Here's how the part is built. I have some questions about the finished solid (model axes, mm). Round coordinates to 2 decimals unless told otherwise and drop trailing zeros. Write each loop counter-clockwise with the first axis right and the second up, starting at its lowest first coordinate (ties: lowest second). Pieces come first, ordered by that corner, then holes. Notation, with made-up numbers: M 17.5,84.5 L 53.5,84.5 A30 ccw 53.5,122.5 Z; hole C -17,80 d4. An arc over 180 degrees is marked long. Use a Markdown table: item, result. Add a question column.
```python
from build123d import *

# Parameters (mm, degrees)
F0_R     = 3.6643363337
F0_R_2   = 12.1990402392
F1_DEPTH = 6.35


# Not quite as in the source:
# - a feature names something its author has since deleted; it is built from what else it names


with BuildPart() as f1:
    # F0 (on Top) → F1 (new body)
    with BuildSketch(Plane.XY):
        Polygon((4.9436837435, 38.7340840895), (-45.8563162565, 38.7340840895), (-45.8563162565, -50.1659159105), (4.9436837435, -50.1659159105), (30.3436837435, -50.1659159105), (55.7436837435, -50.1659159105), (55.7436837435, -5.7159159105), (55.7436837435, 38.7340840895), (30.3436837435, 38.7340840895), align=None)
        with Locations((43.0436837435, -27.9409159105)):
            Circle(F0_R, mode=Mode.SUBTRACT)
        with Locations((-20.4563162565, -5.7159159105)):
            Circle(F0_R_2, mode=Mode.SUBTRACT)
        with Locations((43.0436837435, 16.5090840895)):
            Circle(F0_R, mode=Mode.SUBTRACT)
    extrude(amount=F1_DEPTH)


solid = f1.part
```
Item 1: If we mould it in two halves opening along Y, with no side actions, what happens to faces 1 (the face through (-32.644, -5.18, 3.131)), 2 (the face through (44.735, 13.258, 3.131)), 3 (the face through (6, 38.734, 3)), 4 (the face through (4, -5, 0))? For each: +Y half, -Y half, draft (parallel to the pull), parting line (faces both ways), or undercut.
Item 2: Imagine slicing it at C-C on z = 4. List the corners of the cut face in (x, y) for me.
Item 3: Imagine slicing it at A-A on x = -21. List the corners of the cut face in (y, z) for me.
Item 4: Imagine slicing it at B-B on y = -4. List the corners of the cut face in (x, z) for me, plus the area to 3 significant figures.
Item 5: For pin 1 Ø6.5 at (x, y) = (43.04, 16.51) entering from +Z, with a flat end and sliding along its axis, tell me the tip position at first contact or that it passes through.
Item 6: I need wall thicknesses on probe 1 along X at (y, z) = (-28, 5.25); probe 2 along X at (y, z) = (-8, 6); probe 3 along Y at (x, z) = (-21, 5.25). Which ranges of each line are inside material? Lowest first, please. Write a range as from..to.
The answers:
| question | item | result |
|---|---|---|
| 1 | face 1 | undercut |
| 1 | face 2 | undercut |
| 1 | face 3 | +Y half |
| 1 | face 4 | draft |
| 2 | outline | M -45.86,-50.17 L 55.74,-50.17 L 55.74,38.73 L -45.86,38.73 Z; hole C -20.46,-5.72 d24.4; hole C 43.04,-27.94 d7.33; hole C 43.04,16.51 d7.33 |
| 3 | outline | M -50.17,0 L -17.9,0 L -17.9,6.35 L -50.17,6.35 Z; M 6.47,0 L 38.73,0 L 38.73,6.35 L 6.47,6.35 Z |
| 4 | outline | M -45.86,0 L -32.53,0 L -32.53,6.35 L -45.86,6.35 Z; M -8.38,0 L 55.74,0 L 55.74,6.35 L -8.38,6.35 Z |
| 4 | area | 492 mm² |
| 5 | pin 1 | through |
| 6 | probe 1 | -45.86..39.38, 46.71..55.74 |
| 6 | probe 2 | -45.86..-32.44, -8.47..55.74 |
| 6 | probe 3 | -50.17..-17.9, 6.47..38.73 |
